```python
from build123d import *

# Parameters (mm, degrees)
SKETCH_1_R          = 1.5
EXTRUDE_1_DEPTH     = 15
CUT_EXTRUDE_START   = -11
CUT_EXTRUDE_1_DEPTH = 11
SKETCH_3_W          = 90
SKETCH_3_H          = 57
CUT_EXTRUDE_2_DEPTH = 12
SKETCH_4_R          = 2.8
EXTRUDE_2_DEPTH     = 3.3
EXTRUDE_2_2_DEPTH   = 3.3
EXTRUDE_2_3_DEPTH   = 3.3
EXTRUDE_2_4_DEPTH   = 3.3
SKETCH_5_R          = 1.5
EXTRUDE_3_DEPTH     = 1.3
EXTRUDE_3_2_DEPTH   = 1.3
EXTRUDE_3_3_DEPTH   = 1.3
EXTRUDE_3_4_DEPTH   = 1.3
SKETCH_6_W          = 95
SKETCH_6_H          = 62
CUT_EXTRUDE_3_DEPTH = 5
SKETCH_9_W          = 9.5
SKETCH_9_H          = 2.5
CUT_EXTRUDE_4_DEPTH = 5
CUT_EXTRUDE_5_DEPTH = 73.996164283
FILLET_1_R          = 3
FILLET_3_R          = 1
SKETCH_12_R         = 2.5
EXTRUDE_5_DEPTH     = 3
SKETCH_13_R         = 1.5
CUT_EXTRUDE_6_DEPTH = 73.003055491
CHAMFER_1_SIZE      = 1
SKETCH_15_W         = 82
SKETCH_15_H         = 4
SKETCH_15_W_2       = 2.5
SKETCH_15_H_2       = 20
CUT_EXTRUDE_8_DEPTH = 73.439215899


with BuildPart() as part:
    # 草图1 → 凸台-拉伸1 (new body)
    with BuildSketch(Plane(origin=(0, 0, 0), x_dir=(1, 0, 0), z_dir=(0, 1, 0))):
        with BuildLine():
            Line((-47.5, 31), (-41.5, 31))
            Line((-41.5, 31), (-41.5, 41))
            ThreePointArc((-41.5, 41), (-35.5, 47), (-29.5, 41))
            Line((-29.5, 41), (-29.5, 31))
            Line((-29.5, 31), (-3, 31))
            Line((-3, 31), (-3, 33.8))
            ThreePointArc((-3, 33.8), (0, 36.8), (3, 33.8))
            Line((3, 33.8), (3, 31))
            Line((3, 31), (29.5, 31))
            Line((29.5, 31), (29.5, 41))
            ThreePointArc((29.5, 41), (35.5, 47), (41.5, 41))
            Line((41.5, 41), (41.5, 31))
            Line((41.5, 31), (47.5, 31))
            Line((47.5, 31), (50.8, 31))
            ThreePointArc((50.8, 31), (53.8, 28), (50.8, 25))
            Line((50.8, 25), (47.5, 25))
            Line((47.5, 25), (47.5, -25))
            Line((47.5, -25), (50.8, -25))
            ThreePointArc((50.8, -25), (53.8, -28), (50.8, -31))
            Line((50.8, -31), (47.5, -31))
            Line((47.5, -31), (41.5, -31))
            Line((41.5, -31), (41.5, -41))
            ThreePointArc((41.5, -41), (35.5, -47), (29.5, -41))
            Line((29.5, -41), (29.5, -31))
            Line((29.5, -31), (3, -31))
            Line((3, -31), (3, -33.8))
            ThreePointArc((3, -33.8), (0, -36.8), (-3, -33.8))
            Line((-3, -33.8), (-3, -31))
            Line((-3, -31), (-29.5, -31))
            Line((-29.5, -31), (-29.5, -41))
            ThreePointArc((-29.5, -41), (-35.5, -47), (-41.5, -41))
            Line((-41.5, -41), (-41.5, -31))
            Line((-41.5, -31), (-47.5, -31))
            Line((-47.5, -31), (-50.8, -31))
            ThreePointArc((-50.8, -31), (-53.8, -28), (-50.8, -25))
            Line((-50.8, -25), (-47.5, -25))
            Line((-47.5, -25), (-47.5, 25))
            Line((-47.5, 25), (-50.8, 25))
            ThreePointArc((-50.8, 25), (-53.8, 28), (-50.8, 31))
            Line((-50.8, 31), (-47.5, 31))
        make_face()
        with Locations(Location((-50.8, 28, 0), (0, 0, 270))):
            Circle(SKETCH_1_R, mode=Mode.SUBTRACT)
        with Locations(Location((50.8, 28, 0), (0, 0, 90))):
            Circle(SKETCH_1_R, mode=Mode.SUBTRACT)
        with Locations(Location((50.8, -28, 0), (0, 0, 270))):
            Circle(SKETCH_1_R, mode=Mode.SUBTRACT)
        with Locations(Location((-50.8, -28, 0), (0, 0, 90))):
            Circle(SKETCH_1_R, mode=Mode.SUBTRACT)
        with Locations(Location((0, 33.8, 0), (0, 0, 270))):
            Circle(SKETCH_1_R, mode=Mode.SUBTRACT)
        with Locations(Location((0, -33.8, 0), (0, 0, 90))):
            Circle(SKETCH_1_R, mode=Mode.SUBTRACT)
    extrude(amount=-EXTRUDE_1_DEPTH)

    # 草图2 → 切除-拉伸1 (cut)
    with BuildSketch(Plane.XZ.offset(15).offset(CUT_EXTRUDE_START)):
        with BuildLine():
            Line((-57.023911512, 31), (-3, 31))
            Line((-3, 31), (-3, 33.8))
            ThreePointArc((-3, 33.8), (0, 36.8), (3, 33.8))
            Line((3, 33.8), (3, 31))
            Line((3, 31), (57.023911512, 31))
            Line((57.023911512, 31), (57.023911512, 48.5806389))
            Line((57.023911512, 48.5806389), (-57.023911512, 48.5806389))
            Line((-57.023911512, 48.5806389), (-57.023911512, 31))
        make_face()
        with BuildLine():
            Line((3, -33.8), (3, -31))
            Line((3, -31), (57.023911512, -31))
            Line((57.023911512, -31), (57.023911512, -48.5806389))
            Line((57.023911512, -48.5806389), (-57.023911512, -48.5806389))
            Line((-57.023911512, -48.5806389), (-57.023911512, -31))
            Line((-57.023911512, -31), (-3, -31))
            Line((-3, -31), (-3, -33.8))
            ThreePointArc((-3, -33.8), (0, -36.8), (3, -33.8))
        make_face()
    extrude(amount=CUT_EXTRUDE_1_DEPTH, mode=Mode.SUBTRACT)

    # 草图3 → 切除-拉伸2 (cut)
    with BuildSketch(Plane.XZ.offset(15)):
        Rectangle(SKETCH_3_W, SKETCH_3_H)
    extrude(amount=-CUT_EXTRUDE_2_DEPTH, mode=Mode.SUBTRACT)

    # 草图6 → 切除-拉伸3 (cut)
    with BuildSketch(Plane.XZ.offset(15)):
        Rectangle(SKETCH_6_W, SKETCH_6_H)
    extrude(amount=-CUT_EXTRUDE_3_DEPTH, mode=Mode.SUBTRACT)

    # 草图9 → 切除-拉伸4 (cut)
    with BuildSketch(Plane.XZ.offset(10)):
        with Locations((36.75, 29.75)):
            Rectangle(SKETCH_9_W, SKETCH_9_H)
    extrude(amount=-CUT_EXTRUDE_4_DEPTH, mode=Mode.SUBTRACT)

    # 草图10 → 切除-拉伸5 (cut, through all)
    with BuildSketch(Plane(origin=(0, 0, 0), x_dir=(1, 0, 0), z_dir=(0, 1, 0))):
        with BuildLine():
            Line((-32, -19), (32, -19))
            ThreePointArc((32, -19), (33.414213562, -18.414213562), (34, -17))
            Line((34, -17), (34, 17))
            ThreePointArc((34, 17), (33.414213562, 18.414213562), (32, 19))
            Line((32, 19), (-32, 19))
            ThreePointArc((-32, 19), (-33.414213562, 18.414213562), (-34, 17))
            Line((-34, 17), (-34, -17))
            ThreePointArc((-34, -17), (-33.414213562, -18.414213562), (-32, -19))
        make_face()
    extrude(amount=-CUT_EXTRUDE_5_DEPTH, mode=Mode.SUBTRACT)

    # 圆角1
    fillet_1_edges = [part.edges().sort_by_distance(p)[0] for p in [
        (41.5, -2, -31),
        (29.5, -2, -31),
        (-29.5, -2, -31),
        (-41.5, -2, -31),
        (-41.5, -2, 31),
        (-29.5, -2, 31),
        (29.5, -2, 31),
        (41.5, -2, 31),
    ]]
    fillet(fillet_1_edges, radius=FILLET_1_R)

    # 圆角3
    fillet_3_edges = [part.edges().sort_by_distance(p)[0] for p in [
        (45, -3, 0),
        (0, -3, -28.5),
        (-45, -3, 0),
        (0, -3, 28.5),
        (0, -3, 19),
        (33.414213562, -3, 18.414213562),
        (34, -3, 0),
        (33.414213562, -3, -18.414213562),
        (0, -3, -19),
        (-33.414213562, -3, -18.414213562),
        (-34, -3, 0),
        (-33.414213562, -3, 18.414213562),
    ]]
    fillet(fillet_3_edges, radius=FILLET_3_R)


with BuildPart() as body_2:
    # 草图4 → 凸台-拉伸2 (new body)
    with BuildSketch(Plane.XZ.offset(4)):
        with Locations(Location((-35.5, 41, 0), (0, 0, 270))):
            Circle(SKETCH_4_R)
    extrude(amount=EXTRUDE_2_DEPTH)


with BuildPart() as body_3:
    # 草图4 → Extrude 2 2 (new body)
    with BuildSketch(Plane.XZ.offset(4)):
        with Locations(Location((35.5, 41, 0), (0, 0, 90))):
            Circle(SKETCH_4_R)
    extrude(amount=EXTRUDE_2_2_DEPTH)


with BuildPart() as body_4:
    # 草图4 → Extrude 2 3 (new body)
    with BuildSketch(Plane.XZ.offset(4)):
        with Locations(Location((35.5, -41, 0), (0, 0, 270))):
            Circle(SKETCH_4_R)
    extrude(amount=EXTRUDE_2_3_DEPTH)


with BuildPart() as body_5:
    # 草图4 → Extrude 2 4 (new body)
    with BuildSketch(Plane.XZ.offset(4)):
        with Locations(Location((-35.5, -41, 0), (0, 0, 90))):
            Circle(SKETCH_4_R)
    extrude(amount=EXTRUDE_2_4_DEPTH)


with BuildPart() as body_6:
    # 草图5 → 凸台-拉伸3 (new body)
    with BuildSketch(Plane.XZ.offset(7.3)):
        with Locations(Location((-35.5, 41, 0), (0, 0, 270))):
            Circle(SKETCH_5_R)
    extrude(amount=EXTRUDE_3_DEPTH)


with BuildPart() as body_7:
    # 草图5 → Extrude 3 2 (new body)
    with BuildSketch(Plane.XZ.offset(7.3)):
        with Locations(Location((35.5, 41, 0), (0, 0, 90))):
            Circle(SKETCH_5_R)
    extrude(amount=EXTRUDE_3_2_DEPTH)


with BuildPart() as body_8:
    # 草图5 → Extrude 3 3 (new body)
    with BuildSketch(Plane.XZ.offset(7.3)):
        with Locations(Location((35.5, -41, 0), (0, 0, 270))):
            Circle(SKETCH_5_R)
    extrude(amount=EXTRUDE_3_3_DEPTH)


with BuildPart() as body_9:
    # 草图5 → Extrude 3 4 (new body)
    with BuildSketch(Plane.XZ.offset(7.3)):
        with Locations(Location((-35.5, -41, 0), (0, 0, 90))):
            Circle(SKETCH_5_R)
    extrude(amount=EXTRUDE_3_4_DEPTH)


with BuildPart() as body_4_1:
    add(body_4.part)

    # Combine 1: union part, body 8, body 2, body 5, body 6, body 9, body 3, body 7
    add(part.part)
    add(body_8.part)
    add(body_2.part)
    add(body_5.part)
    add(body_6.part)
    add(body_9.part)
    add(body_3.part)
    add(body_7.part)

    # 草图12 → 凸台-拉伸5 (add)
    with BuildSketch(Plane.XZ.offset(3)):
        with Locations(Location((-39.5, 15, 0), (0, 0, 90))):
            Circle(SKETCH_12_R)
        with Locations(Location((-39.5, -15, 0), (0, 0, 90))):
            Circle(SKETCH_12_R)
        with Locations(Location((39.5, -15, 0), (0, 0, 90))):
            Circle(SKETCH_12_R)
        with Locations(Location((39.5, 15, 0), (0, 0, 90))):
            Circle(SKETCH_12_R)
    extrude(amount=EXTRUDE_5_DEPTH)

    # 草图13 → 切除-拉伸6 (cut, through all)
    with BuildSketch(Plane.XZ.offset(6)):
        with Locations(Location((39.5, -15, 0), (0, 0, 270))):
            Circle(SKETCH_13_R)
        with Locations(Location((39.5, 15, 0), (0, 0, 270))):
            Circle(SKETCH_13_R)
        with Locations(Location((-39.5, -15, 0), (0, 0, 270))):
            Circle(SKETCH_13_R)
        with Locations(Location((-39.5, 15, 0), (0, 0, 270))):
            Circle(SKETCH_13_R)
    extrude(amount=-CUT_EXTRUDE_6_DEPTH, mode=Mode.SUBTRACT)

    # 倒角1
    chamfer_1_edges = [body_4_1.edges().sort_by_distance(p)[0] for p in [
        (39.5, 0, 16.5),
        (-39.5, 0, -13.5),
        (-39.5, 0, 16.5),
        (39.5, 0, -13.5),
    ]]
    chamfer(chamfer_1_edges, length=CHAMFER_1_SIZE)

    # 草图15 → 切除-拉伸8 (cut, through all)
    with BuildSketch(Plane.XZ.offset(3)):
        with Locations((0, 23.5)):
            Rectangle(SKETCH_15_W, SKETCH_15_H)
        with Locations((0, -23.5)):
            Rectangle(SKETCH_15_W, SKETCH_15_H)
        with Locations((-39.5, 0)):
            Rectangle(SKETCH_15_W_2, SKETCH_15_H_2)
        with Locations((39.5, 0)):
            Rectangle(SKETCH_15_W_2, SKETCH_15_H_2)
    extrude(amount=-CUT_EXTRUDE_8_DEPTH, mode=Mode.SUBTRACT)


solid = body_4_1.part
```
The listing builds one solid part. Answer for the finished solid, in the listing's coordinates (mm). A direction names the side the tool comes from. Round coordinates to 2 decimals unless told otherwise and drop trailing zeros. Loops run counter-clockwise (first coordinate to the right, second up) from the corner with the lowest first, then second, coordinate; pieces in that order, holes last.
1) A cutting plane is placed at B-B on x = -23. Determine the outline of the cut face in (y, z), plus the area to 3 significant figures.
Outcome:
outline: (-10, -31) - (0, -31) - (0, -25.5) - (-3, -25.5) - (-3, -27.5) arc R1 cw to (-4, -28.5) - (-10, -28.5) - close; (-10, 28.5) - (-4, 28.5) arc R1 cw to (-3, 27.5) - (-3, 25.5) - (0, 25.5) - (0, 31) - (-10, 31) - close; (-3, -21.5) - (0, -21.5) - (0, -19) - (-2, -19) arc R1 ccw to (-3, -20) - close; (-3, 20) arc R1 ccw to (-2, 19) - (0, 19) - (0, 21.5) - (-3, 21.5) - close
area: 83.0 mm2
2) For faces 1 (the face through (-0.1, -7.4, -36.8)), 2 (the face through (-49, -7, -25)), 3 (the face through (32.767, -5.627, -40.393)), 4 (the face through (49, -7, -25)), 5 (the face through (-41, -2, -24)), determine the directions among +Z, -Z, +X, -X, +Y, -Y from which every point of the face is accessible in a straight line to the end or side of a thin tool.
Outcome:
face 1: -Z, +Y, -Y
face 2: -X, +Y, -Y
face 3: -Y
face 4: +X, +Y, -Y
face 5: +Y, -Y
3) A cutting plane is placed at A-A on y = -13. Give the number of separate pieces and of enclosed holes in the cut face, plus the area to 3 significant figures.
Outcome:
separate pieces: 6
enclosed holes: 6
area: 155 mm2
4) Given P1, Ø6, axis at y = -10.5, z = 12, coming from the -X side; P2, Ø2, axis at x = -19.5, y = -1.5, coming from the -Z side; P3, Ø0.8, axis at y = -9, z = -33, coming from the -X side, each flat-ended and moving along its own axis, determine where each tip first touches the part or whether it passes through.
Outcome:
P1: stops at x = -47.5
P2: stops at z = -31
P3: stops at x = -3
5) For a pull along Z with two mould halves and no side action, classify faces 6 (the face through (28.6, -2.03, 31.86)), 7 (the face through (-35.6, -2, -47)), 8 (the face through (41.5, -2, 37)), 9 (the face through (0, -13, -31)) as released by +Z, released by -Z, zero draft, split by the parting line, or undercut.
Outcome:
face 6: released by +Z
face 7: released by -Z
face 8: zero draft
face 9: undercut
6) Consider line 1 (X direction, y = -0.75, z = -1.5); line 2 (X direction, y = -2.05, z = -15); line 3 (X direction, y = -5.5, z = -33.8). Determine where each line is inside the solid, lowest interval first.
Outcome:
line 1: x = -47.5 to -40.75, -38.25 to -34, 34 to 38.25, 40.75 to 47.5
line 2: x = -47.5 to -41, -38 to -34, 34 to 38, 41 to 47.5
line 3: x = -3 to -1.5, 1.5 to 3
